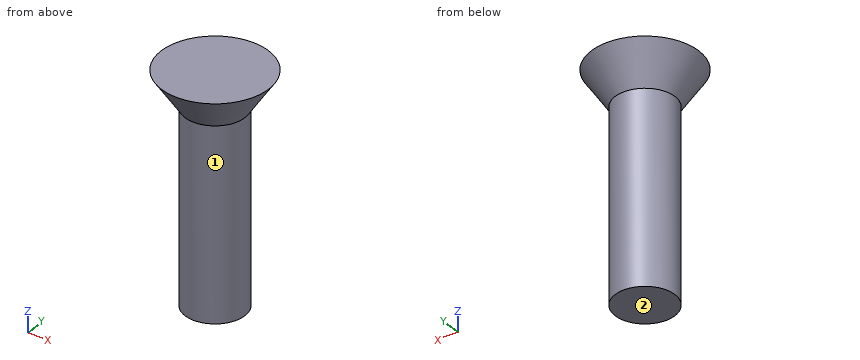
from build123d import *

# Parameters (mm, degrees)
CYLINDER011_R                   = 2.5
CYLINDER011_DEPTH               = 16
FUSION001018017_PLACEMENT_ANGLE = 180


with BuildPart() as cone003:
    # Cone003 → Cone003 (revolve)
    with BuildSketch(Plane(origin=(0, 0, -3), x_dir=(1, 0, 0), z_dir=(0, -1, 0))):
        Polygon((0, 0), (4.5, 0), (2.5, 3), (0, 3), align=None)
    revolve(axis=Axis((0, 0, -3), (0, 0, 1)))


with BuildPart() as obj1:
    # Cylinder011 → Cylinder011 (new body)
    with BuildSketch(Plane.XY):
        Circle(CYLINDER011_R)
    extrude(amount=CYLINDER011_DEPTH)

    # Fusion001018017: union Cone003
    add(cone003.part)


with BuildPart() as obj1_1:
    # Fusion001018017 placement: moved
    add(obj1.part.moved(Location((45, 15, 21))).rotate(Axis((45, 15, 21), (0, 1, 0)), FUSION001018017_PLACEMENT_ANGLE))


solid = obj1_1.part
Could you check a few things on this model? Use its own coordinates, in mm. Face numbers are marked on the shaded views. A direction names the side the tool comes from. Coordinates: 2 decimals unless noted, no trailing zeros. Write each loop counter-clockwise with the first axis right and the second up, starting at its lowest first coordinate (ties: lowest second). Pieces come first, ordered by that corner, then holes. Notation, with made-up numbers: M 88.25,36.5 L 120.25,36.5 A12 ccw 120.25,48.5 Z; hole C -27.5,40 d8. An arc over 180 degrees is marked long. One line per question, with ' | ' between items.
1) For the marked faces 1 and 2, which set-ups out of +Z, -Z, +X, -X, +Y, -Y let a thin tool reach every point of the face, with its end or its side?
Checks:
face 1: -Z | face 2: -Z, +X, -X, +Y, -Y
2) Imagine slicing it at A-A, the plane x = 45. Write out the boundary of the cut face in (y, z).
Checks:
outline: M 10.5,24 L 12.5,21 L 12.5,5 L 17.5,5 L 17.5,21 L 19.5,24 Z
3) Imagine slicing it at C-C, the plane z = 19.75. Write out the boundary of the cut face in (x, y).
Checks:
outline: C 45,15 d5
4) For pin 1 Ø4 at (y, z) = (18, 18.5) entering from -X; pin 2 Ø5 at (y, z) = (14.5, 8) entering from -X; pin 3 Ø5 at (x, z) = (48.5, 17.5) entering from +Y, each with a flat end and sliding along its axis, tell me the tip position at first contact or that it passes through.
Checks:
pin 1: x = 42.71 | pin 2: x = 42.5 | pin 3: y = 17.29
5) I need wall thicknesses on probe 1 along Y at (x, z) = (44.75, 14.5); probe 2 along Z at (x, y) = (42, 14.75); probe 3 along Y at (x, z) = (44, 13.75). Which ranges of each line are inside material? Lowest first, please. Write a range as [from, to].
Checks:
probe 1: [12.51, 17.49] | probe 2: [21.77, 24] | probe 3: [12.71, 17.29]
6) Imagine slicing it at B-B, the plane y = 15. Write out the boundary of the cut face in (x, z), and give its area (3 significant figures).
Checks:
outline: M 40.5,24 L 42.5,21 L 42.5,5 L 47.5,5 L 47.5,21 L 49.5,24 Z | area: 101 mm²
